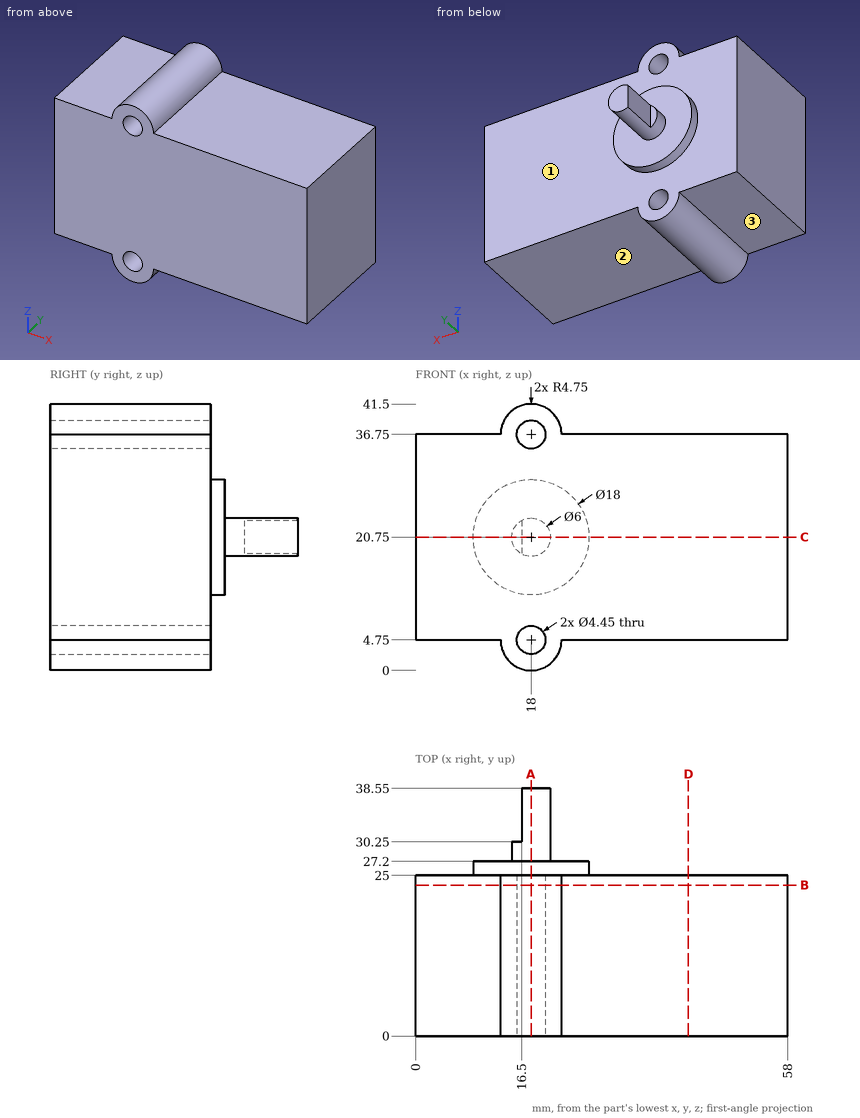
Design review of the part shown in the three views and the two pictorial views. Dimensions are in mm from the part's minimum x, y and z. A direction names the side the tool comes from. Give positions to 0.01 mm unless a question says otherwise; leave off trailing zeros. Loops run counter-clockwise (first coordinate to the right, second up) from the corner with the lowest first, then second, coordinate; pieces in that order, holes last. Notation, with made-up numbers: (50, 22.25) - (54, 22.25) arc R19 cw to (54, 38.25) - close; hole circle Ø7 at (-27.75, 40.5). An arc over 180 degrees is marked (long way). Answer as a JSON object with one key per item and string values.
Q1. Add section A-A on x = 18. State the section outline as (y, z) points (3 decimals).
Worked out:
{"outline": "(0, 0) - (25, 0) - (25, 2.525) - (0, 2.525) - close; (0, 6.975) - (25, 6.975) - (25, 11.75) - (27.2, 11.75) - (27.2, 17.75) - (38.55, 17.75) - (38.55, 23.75) - (27.2, 23.75) - (27.2, 29.75) - (25, 29.75) - (25, 34.525) - (0, 34.525) - close; (0, 38.975) - (25, 38.975) - (25, 41.5) - (0, 41.5) - close"}
Q2. Add section D-D on x = 42.5. State the section outline as (y, z) points, plus the area to 3 significant figures.
Worked out:
{"outline": "(0, 4.75) - (25, 4.75) - (25, 36.75) - (0, 36.75) - close", "area": "800 mm^2"}
Q3. Add section B-B on y = 23.5. State the section outline as (x, z) points (3 decimals).
Worked out:
{"outline": "(0, 4.75) - (13.25, 4.75) arc R4.75 ccw to (22.75, 4.75) - (58, 4.75) - (58, 36.75) - (22.75, 36.75) arc R4.75 ccw to (13.25, 36.75) - (0, 36.75) - close; hole circle Ø4.45 at (18, 4.75); hole circle Ø4.45 at (18, 36.75)"}
Q4. Insertion check: pin 1 (1.6 mm diameter, centred on y = 34, z = 19.5, fed in from -X); pin 2 (4 mm diameter, centred on x = 27, z = 6.5, fed in from +Y); pin 3 (7.5 mm diameter, centred on x = 47, y = 15.5, fed in from -Z); pin 4 (2.5 mm diameter, centred on x = 18, z = 4.75, fed in from +Y). Each pin has a flat end and moves straight along its axis. Give the tip position at first contact, or say it passes through.
Worked out:
{"pin 1": "stops at x = 16.5", "pin 2": "stops at y = 25", "pin 3": "stops at z = 4.75", "pin 4": "passes through"}
Q5. Add section C-C on z = 20.75. State the section outline as (x, y) points, plus the area to 3 significant figures.
Worked out:
{"outline": "(0, 0) - (58, 0) - (58, 25) - (27, 25) - (27, 27.2) - (21, 27.2) - (21, 38.55) - (16.5, 38.55) - (16.5, 30.25) - (15, 30.25) - (15, 27.2) - (9, 27.2) - (9, 25) - (0, 25) - close", "area": "1,550 mm^2"}
Q6. For the marked faces 1, 2 and 3, list the 3-axis set-ups (+Z, -Z, +X, -X, +Y, -Y) from which the entire face can be reached by the end or side of a thin tool; tool diameter is ignored.
Worked out:
{"face 1": "+Y", "face 2": "-Z, +X, +Y, -Y", "face 3": "-Z, -X, +Y, -Y"}
Q7. To check wall thickness, follow line 1 along Z through (x, y) = (54, 13); line 2 along Y through (x, z) = (3, 6); line 3 along Z through (x, y) = (16.5, 24). State the ranges of each line that lie inside material, in increasing order.
Worked out:
{"line 1": "z = 4.75 to 36.75", "line 2": "y = 0 to 25", "line 3": "z = 0.24 to 3.11, 6.39 to 35.11, 38.39 to 41.26"}
